from build123d import *

# Parameters (mm, degrees)
RESSALTO_EXTRUS_O1_DEPTH = 3


with BuildPart() as part:
    # Esboço1 → Ressalto-extrusão1 (new body)
    with BuildSketch(Plane.XY):
        Polygon((0, 0), (2.25, 0), (2.25, -4), (1, -4), (1, -6.5), (2.25, -6.5), (2.25, -9), (5.25, -9), (5.25, -6.5), (6.5, -6.5), (6.5, -4), (5.25, -4), (5.25, 0), (7.5, 0), (7.5, 5), (13.5, 5), (13.5, 0), (13.5, -35), (13.5, -40), (7.5, -40), (7.5, -35), (5.25, -35), (5.25, -31), (6.5, -31), (6.5, -28.5), (5.25, -28.5), (5.25, -26), (2.25, -26), (2.25, -28.5), (1, -28.5), (1, -31), (2.25, -31), (2.25, -35), (0, -35), (0, -40), (-6, -40), (-6, -35), (-6, 0), (-6, 5), (0, 5), align=None)
    extrude(amount=RESSALTO_EXTRUS_O1_DEPTH)


solid = part.part
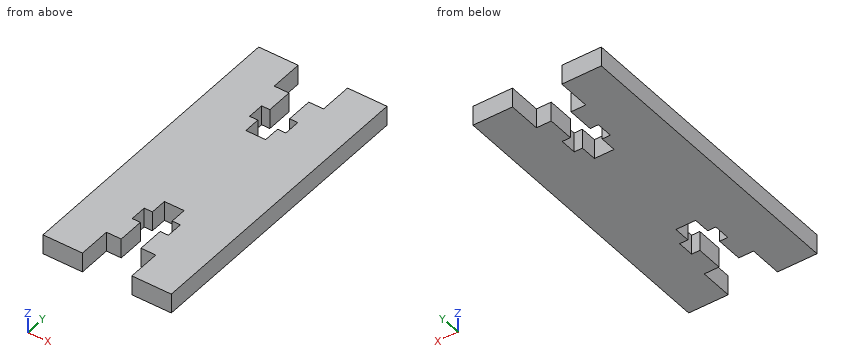
Can you work these out from the model? Positions are in its coordinate system, mm. Round coordinates to 2 decimals unless told otherwise and drop trailing zeros. Write each loop counter-clockwise with the first axis right and the second up, starting at its lowest first coordinate (ties: lowest second). Pieces come first, ordered by that corner, then holes. Notation, with made-up numbers: (30, -11) -> (86, -11) arc R21 ccw to (86, 8) -> close; hole circle Ø4 at (48, 79.5). An arc over 180 degrees is marked (long way). Use one line per item in the form item = value. Start each with the question number.
Q1. I'm going to push flat-ended pins straight in: P1, Ø1, axis at x = 2, z = 1.5, coming from the -Y side; P2, Ø1, axis at x = 6, z = 1, coming from the +Y side. Where does each tip first touch, or does it pass through?
Q2. Imagine slicing it at C-C (x = 4). Please give me the cut outline in (y, z).
Q3. If I drill on probe 1 along Y at (x, z) = (6, 1.5); probe 2 along X at (y, z) = (-8, 2.15); probe 3 along X at (y, z) = (-30, 0.1), over which ranges is the centre line in solid material (lowest first)? Write a range as [from, to].
Q4. Imagine slicing it at B-B (x = 1.75). Please give me the cut outline in (y, z), then the cut area to 3 significant figures.
Q5. Imagine slicing it at A-A (y = -36). Please give me the cut outline in (x, z), then the cut area to 3 significant figures.
Worked out:
q1.P1 = -35
q1.P2 = 0
q2.outline = (-26, 0) -> (-9, 0) -> (-9, 3) -> (-26, 3) -> close
q3.probe_1 = [-35, -31], [-28.5, -6.5], [-4, 0]
q3.probe_2 = [-6, 2.25], [5.25, 13.5]
q3.probe_3 = [-6, 1], [6.5, 13.5]
q4.outline = (-35, 0) -> (-31, 0) -> (-31, 3) -> (-35, 3) -> close; (-28.5, 0) -> (-6.5, 0) -> (-6.5, 3) -> (-28.5, 3) -> close; (-4, 0) -> (0, 0) -> (0, 3) -> (-4, 3) -> close
q4.area = 90.0 mm^2
q5.outline = (-6, 0) -> (0, 0) -> (0, 3) -> (-6, 3) -> close; (7.5, 0) -> (13.5, 0) -> (13.5, 3) -> (7.5, 3) -> close
q5.area = 36.0 mm^2
